```python
from build123d import *

# Parameters (mm, degrees)
F1_DEPTH = 203.2


with BuildPart() as f1:
    # F0 (on Front) → F1 (new body)
    with BuildSketch(Plane.XZ):
        with BuildLine():
            ThreePointArc((0, -41.275), (-41.275, 0), (0, 41.275))
            Line((0, 41.275), (25.92662, 41.275))
            Line((25.92662, 41.275), (25.92662, 44.45))
            Line((25.92662, 44.45), (0, 44.45))
            ThreePointArc((0, 44.45), (-44.45, 0), (0, -44.45))
            Line((0, -44.45), (0, -41.275))
        make_face()
    extrude(amount=F1_DEPTH)


solid = f1.part
```
For this review, take the finished solid that the model builds, in its own axes (mm). Coordinates: 2 decimals unless noted, no trailing zeros. Write each loop counter-clockwise with the first axis right and the second up, starting at its lowest first coordinate (ties: lowest second). Pieces come first, ordered by that corner, then holes. Notation, with made-up numbers: (29, 48.25) - (62, 48.25) arc R29 cw to (62, 80.25) - close; hole circle Ø10 at (71, 78.25). An arc over 180 degrees is marked (long way). Answer in a Markdown table with one row per item. Add a question column.
Q1. We need section A-A, the plane x = -26.5. State the section outline as (y, z) points, and give its area (3 significant figures).
Q2. We need section B-B, the plane y = -22.5. State the section outline as (x, z) points (3 decimals).
Q3. We need section C-C, the plane x = -18. State the section outline as (y, z) points, and give its area (3 significant figures).
Q4. We need section D-D, the plane z = 0. State the section outline as (x, y) points (3 decimals), and give its area (3 significant figures).
Q5. For probe 1 along Z at (x, y) = (4, -80) (3 decimals); probe 2 along X at (y, z) = (-184.5, 0) (3 decimals); probe 3 along Z at (x, y) = (-0.5, -119), list the stretches that pass through material, from the lowest coordinate up.
Q6. Draft analysis for pull direction Z (two halves, no side actions). For faces 1 (the flat face through (13, -100, 44.45)), 2 (the cylindrical face through (-41.265, -100.178, -0.908)), 3 (the flat face through (13, -100, 41.275)), state which applies: +Z half, -Z half, draft (parallel to the pull), parting line (faces both ways), or undercut.
Q7. For P1, Ø1.6, axis at y = -52.5, z = -43.5, coming from the +X side; P2, Ø5, axis at x = -27, y = -183, coming from the -Z side; P3, Ø12, axis at x = -2, y = -173.5, coming from the -Z side; P4, Ø5, axis at y = -145, z = -25.5, coming from the -X side, all flat-tipped, find the tip position at first contact; note any pin that passes through.
Answer list:
| question | item | result |
|---|---|---|
| 1 | outline | (-203.2, -35.69) - (0, -35.69) - (0, -31.64) - (-203.2, -31.64) - close; (-203.2, 31.64) - (0, 31.64) - (0, 35.69) - (-203.2, 35.69) - close |
| 1 | area | 1,640 mm2 |
| 2 | outline | (0, -44.45) - (0, -41.275) arc R41.275 cw to (0, 41.275) - (25.927, 41.275) - (25.927, 44.45) - (0, 44.45) arc R44.45 ccw to start |
| 3 | outline | (-203.2, -40.64) - (0, -40.64) - (0, -37.14) - (-203.2, -37.14) - close; (-203.2, 37.14) - (0, 37.14) - (0, 40.64) - (-203.2, 40.64) - close |
| 3 | area | 1,420 mm2 |
| 4 | outline | (-44.45, -203.2) - (-41.275, -203.2) - (-41.275, 0) - (-44.45, 0) - close |
| 4 | area | 645 mm2 |
| 5 | probe 1 | z = 41.275 to 44.45 |
| 5 | probe 2 | x = -44.45 to -41.275 |
| 5 | probe 3 | z = -44.45 to -41.27, 41.27 to 44.45 |
| 6 | face 1 | +Z half |
| 6 | face 2 | undercut |
| 6 | face 3 | -Z half |
| 7 | P1 | stops at x = 0 |
| 7 | P2 | stops at z = -37.09 |
| 7 | P3 | stops at z = -44.45 |
| 7 | P4 | stops at x = -38.04 |
